from build123d import *

# Parameters (mm, degrees)
SKETCH_4_R          = 100
SKETCH_4_W          = 23
SKETCH_4_H          = 39
CUT_EXTRUDE_1_DEPTH = 8


with BuildPart() as part:
    # ｽｹｯﾁ1 → 回転1 (revolve)
    with BuildSketch(Plane.XY, mode=Mode.PRIVATE) as revolve_1_sk:
        Polygon((-28, 8.5), (-22, 8.5), (-22, 6.5), (-6, 6.5), (-6, 8.5), (0, 8.5), (0, 19.5), (-8, 19.5), (-8, 10.5), (-28, 10.5), align=None)
    revolve(revolve_1_sk.sketch.rotate(Axis((0, 0, 0), (-1, 0, 0)), 270), axis=Axis((0, 0, 0), (-1, 0, 0)))

    # ｽｹｯﾁ2 → ｶｯﾄ - 回転1 (revolve, cut)
    with BuildSketch(Plane.XY, mode=Mode.PRIVATE) as cut_revolve_1_sk:
        Polygon((-8, 14.5), (-8, 16.75), (-4.1, 16.75), (-4.1, 18.5), (0, 18.5), (0, 14.5), align=None)
    revolve(cut_revolve_1_sk.sketch.rotate(Axis((0, 14.5, 0), (-1, 0, 0)), 270), axis=Axis((0, 14.5, 0), (-1, 0, 0)), mode=Mode.SUBTRACT)

    # ｽｹｯﾁ3 → ｶｯﾄ - 回転2 (revolve, cut)
    with BuildSketch(Plane.XY, mode=Mode.PRIVATE) as cut_revolve_2_sk:
        Polygon((-8, -14.5), (-8, -12.25), (-4.1, -12.25), (-4.1, -10.5), (0, -10.5), (0, -14.5), align=None)
    revolve(cut_revolve_2_sk.sketch.rotate(Axis((0, -14.5, 0), (-1, 0, 0)), 270), axis=Axis((0, -14.5, 0), (-1, 0, 0)), mode=Mode.SUBTRACT)

    # ｽｹｯﾁ4 → ｶｯﾄ - 押し出し1 (cut)
    with BuildSketch(Plane(origin=(0, 0, 0), x_dir=(0, 0, -1), z_dir=(1, 0, 0))):
        Circle(SKETCH_4_R)
        Rectangle(SKETCH_4_W, SKETCH_4_H, mode=Mode.SUBTRACT)
    extrude(amount=-CUT_EXTRUDE_1_DEPTH, mode=Mode.SUBTRACT)


solid = part.part
CAD build for the part. Positions are in the model's coordinates, mm. A direction names the side the tool comes from. Round coordinates to 2 decimals unless told otherwise and drop trailing zeros. Write each loop counter-clockwise with the first axis right and the second up, starting at its lowest first coordinate (ties: lowest second). Pieces come first, ordered by that corner, then holes.
(1) Slice it at A-A, the plane y = 0. Write the cut outline in (x, z).
(2) 3-axis set-ups, long thin cutter, end or side, ignore diameter. For faces 1 (the face through (-4.1, 13, -2)), 2 (the face through (-18.1, 3.2, 10)), 3 (the face through (-6.023, -16.696, -0.488)): which of +Z, -Z, +X, -X, +Y, -Y reach the whole face in a straight line?
(3) Probe line 1 along Y through (x, z) = (-5.85, 0); line 2 along Y through (x, z) = (-3, -1.25); line 3 along Y through (x, z) = (-16.5, 0). List the from-to ranges inside material, lowest first.
(4) Slice it at B-B, the plane x = -5.25. Write the cut outline in (y, z).
(5) Drop flat-ended pins along their axis: P1, Ø2.5, axis at y = -16, z = -1.5, coming from the +X side; P2, Ø5, axis at y = 5.5, z = 0, coming from the -X side; P3, Ø12, axis at y = 14, z = -1.5, coming from the +X side; P4, Ø2, axis at x = -9.5, z = 5, coming from the -Y side. Give the stop position or say it passes through.
(6) Slice it at C-C, the plane z = 0. Count the separate pieces of the cut face and the enclosed holes in it, and give its area (3 significant figures).
(7) Slice it at D-D, the plane x = -10.75. Write the cut outline in (y, z).
From the geometry:
1. outline: (-28, -10.5) - (-8, -10.5) - (-8, -11.5) - (0, -11.5) - (0, -8.5) - (-6, -8.5) - (-6, -6.5) - (-22, -6.5) - (-22, -8.5) - (-28, -8.5) - close; (-28, 8.5) - (-22, 8.5) - (-22, 6.5) - (-6, 6.5) - (-6, 8.5) - (0, 8.5) - (0, 11.5) - (-8, 11.5) - (-8, 10.5) - (-28, 10.5) - close
2. face 1: +X
2. face 2: -X
2. face 3: +X, -X
3. line 1: y = -19.5 to -16.75, -12.25 to -8.5, 8.5 to 12.25, 16.75 to 19.5
3. line 2: y = -19.46 to -18.3, -10.7 to -8.41, 8.41 to 10.7, 18.3 to 19.46
3. line 3: y = -10.5 to -6.5, 6.5 to 10.5
4. outline: (-15.75, -11.5) - (15.75, -11.5) arc R19.5 ccw to (15.75, 11.5) - (-15.75, 11.5) arc R19.5 ccw to start; hole circle Ø4.5 at (-14.5, 0); hole circle Ø17 at (0, 0); hole circle Ø4.5 at (14.5, 0)
5. P1: stops at x = -4.1
5. P2: stops at x = -22
5. P3: stops at x = 0
5. P4: stops at y = -9.71
6. separate pieces: 4
6. enclosed holes: 0
6. area: 219 mm2
7. outline: circle Ø21 at (0, 0); hole circle Ø13 at (0, 0)
